Part model, mm, in its own coordinate system. A direction names the side the tool comes from. Coordinates: 2 decimals unless noted, no trailing zeros. Loops run counter-clockwise (first coordinate to the right, second up) from the corner with the lowest first, then second, coordinate; pieces in that order, holes last. Notation, with made-up numbers: (26.25, 13.25) - (68.25, 13.25) arc R10 ccw to (68.25, 31.25) - close; hole circle Ø9 at (68, 34). An arc over 180 degrees is marked (long way). Use a Markdown table: item, result. Add a question column.
1) Band-saw the part on C-C (x = -1). Give the cut face in (y, z).
2) Tool access for faces 1 (the face through (0, 0, 2.5)), 2 (the face through (-5.5, 10, -8.2)), 3 (the face through (5.4, -7.5, -7.8)), 4 (the face through (-3.134, -8.732, -12.928)), 5 (the face through (5.4, -10, -7.8)): list every direction of +Z, -Z, +X, -X, +Y, -Y with a clear straight run to the whole face (end or side of a thin tool).
3) Drop flat-ended pins along their axis: P1, Ø8.5, axis at x = -4.5, z = -7, coming from the +Y side; P2, Ø6, axis at y = -7, z = -12, coming from the -X side; P3, Ø1, axis at x = -5.5, z = -5, coming from the -Y side; P4, Ø2.5, axis at x = 3, z = -9.5, coming from the +Y side. Give the stop position or say it passes through.
4) Probe probe 1 along Y at (x, z) = (4.75, -5); probe 2 along Z at (x, y) = (-7, 4.75); probe 3 along X at (y, z) = (7.75, -9.25). List the from-to ranges inside material, lowest first. Write a range as [from, to].
5) Band-saw the part on A-A (x = 6). Give the cut face in (y, z), plus the area to 3 significant figures.
6) Band-saw the part on B-B (z = -9). Give the cut face in (x, y).
7) Band-saw the part on D-D (y = 8.75). Give the cut face in (x, z).
8) Pull direction Y, two halves, no side cores. Call faces 6 (the face through (-5.5, -10, -8.2)), 7 (the face through (-5.5, -7.5, -8.2)), 8 (the face through (-3.134, 8.732, -12.928)), 9 (the face through (0, 0, -2.5)): +Y half, -Y half, draft (parallel to the pull), parting line (faces both ways), or undercut.
from build123d import *

# Parameters (mm, degrees)
F1_DEPTH = 12.5
F2_START = 7.5
F2_DEPTH = 2.5
F3_START = -7.5
F3_DEPTH = 2.5


with BuildPart() as f1:
    # F0 (on Front) → F1 (new body, symmetric)
    with BuildSketch(Plane.XZ):
        with BuildLine():
            Line((7.5, 2.5), (-7.5, 2.5))
            Line((-7.5, 2.5), (-7.5, -2.5))
            Line((-7.5, -2.5), (-5.5901699437, -2.5))
            ThreePointArc((-5.5901699437, -2.5), (0, 0), (5.5901699437, -2.5))
            Line((5.5901699437, -2.5), (7.5, -2.5))
            Line((7.5, -2.5), (7.5, 2.5))
        make_face()
        with BuildLine():
            ThreePointArc((5.5901699437, -2.5), (0, 0), (-5.5901699437, -2.5))
            Line((-5.5901699437, -2.5), (0, -2.5))
            Line((0, -2.5), (5.5901699437, -2.5))
        make_face()
    extrude(amount=F1_DEPTH, both=True)

    # F0 (on Front) → F2 (join)
    with BuildSketch(Plane.XZ.offset(F2_START)):
        with BuildLine():
            Line((0, -2.5), (-5.5901699437, -2.5))
            ThreePointArc((-5.5901699437, -2.5), (-7.4057102945, -8.6855188883), (-3.75, -13.9951905284))
            Line((-3.75, -13.9951905284), (-2.5, -11.8301270189))
            ThreePointArc((-2.5, -11.8301270189), (-4.8296291314, -6.2059047745), (0, -2.5))
        make_face()
        with BuildLine():
            ThreePointArc((7.5, -7.5), (7.0062926922, -4.8238343267), (5.5901699437, -2.5))
            Line((5.5901699437, -2.5), (0, -2.5))
            ThreePointArc((0, -2.5), (3.5355339059, -3.9644660941), (5, -7.5))
            ThreePointArc((5, -7.5), (4.3301270189, -10), (2.5, -11.8301270189))
            Line((2.5, -11.8301270189), (3.75, -13.9951905284))
            ThreePointArc((3.75, -13.9951905284), (6.4951905284, -11.25), (7.5, -7.5))
        make_face()
    extrude(amount=F2_DEPTH)

    # F0 (on Front) → F3 (join)
    with BuildSketch(Plane.XZ.offset(F3_START)):
        with BuildLine():
            ThreePointArc((7.5, -7.5), (7.0062926922, -4.8238343267), (5.5901699437, -2.5))
            Line((5.5901699437, -2.5), (0, -2.5))
            ThreePointArc((0, -2.5), (3.5355339059, -3.9644660941), (5, -7.5))
            ThreePointArc((5, -7.5), (4.3301270189, -10), (2.5, -11.8301270189))
            Line((2.5, -11.8301270189), (3.75, -13.9951905284))
            ThreePointArc((3.75, -13.9951905284), (6.4951905284, -11.25), (7.5, -7.5))
        make_face()
        with BuildLine():
            Line((0, -2.5), (-5.5901699437, -2.5))
            ThreePointArc((-5.5901699437, -2.5), (-7.4057102945, -8.6855188883), (-3.75, -13.9951905284))
            Line((-3.75, -13.9951905284), (-2.5, -11.8301270189))
            ThreePointArc((-2.5, -11.8301270189), (-4.8296291314, -6.2059047745), (0, -2.5))
        make_face()
    extrude(amount=-F3_DEPTH)


solid = f1.part
Answer block:
| question | item | result |
|---|---|---|
| 1 | outline | (-12.5, -2.5) - (-10, -2.5) - (-10, -2.6) - (-7.5, -2.6) - (-7.5, -2.5) - (7.5, -2.5) - (7.5, -2.6) - (10, -2.6) - (10, -2.5) - (12.5, -2.5) - (12.5, 2.5) - (-12.5, 2.5) - close |
| 2 | face 1 | +Z, +X, -X, +Y, -Y |
| 2 | face 2 | -Z, +X, -X, +Y |
| 2 | face 3 | -Z, +X, -X |
| 2 | face 4 | -Z, +Y, -Y |
| 2 | face 5 | -Z, +X, -X, -Y |
| 3 | P1 | y = 10 |
| 3 | P2 | x = -7.34 |
| 3 | P3 | y = -10 |
| 3 | P4 | through |
| 4 | probe 1 | [-10, -7.5], [7.5, 10] |
| 4 | probe 2 | [-2.5, 2.5] |
| 4 | probe 3 | [-7.29, -4.68], [4.68, 7.29] |
| 5 | outline | (-12.5, -2.5) - (12.5, -2.5) - (12.5, 2.5) - (-12.5, 2.5) - close; (-10, -12) - (-7.5, -12) - (-7.5, -3) - (-10, -3) - close; (7.5, -12) - (10, -12) - (10, -3) - (7.5, -3) - close |
| 5 | area | 170 mm2 |
| 6 | outline | (-7.35, -10) - (-4.77, -10) - (-4.77, -7.5) - (-7.35, -7.5) - close; (-7.35, 7.5) - (-4.77, 7.5) - (-4.77, 10) - (-7.35, 10) - close; (4.77, -10) - (7.35, -10) - (7.35, -7.5) - (4.77, -7.5) - close; (4.77, 7.5) - (7.35, 7.5) - (7.35, 10) - (4.77, 10) - close |
| 7 | outline | (-7.5, -2.5) - (-5.59, -2.5) arc R7.5 ccw to (-3.75, -14) - (-2.5, -11.83) arc R5 cw (long way) to (2.5, -11.83) - (3.75, -14) arc R7.5 ccw to (5.59, -2.5) - (7.5, -2.5) - (7.5, 2.5) - (-7.5, 2.5) - close |
| 8 | face 6 | -Y half |
| 8 | face 7 | undercut |
| 8 | face 8 | draft |
| 8 | face 9 | undercut |
